```python
from build123d import *

# Parameters (mm, degrees)
F1_W          = 40
F1_H          = 40
F1_R          = 1.7
F2_DEPTH      = 3
F0_W          = 29.764212
F0_H          = 22.853858
F3_DEPTH      = 15
F0_W_2        = 24.935725
F0_H_2        = 6.393774
F4_DEPTH      = 3
F5_R          = 10
F7_DEPTH      = 25
F7_DEPTH_BACK = 25


with BuildPart() as f2:
    # F1 (on Front) → F2 (new body)
    with BuildSketch(Plane.XZ):
        Rectangle(F1_W, F1_H)
        with Locations((-16.410692, -16.77718)):
            Circle(F1_R, mode=Mode.SUBTRACT)
        with Locations((16.730379, -16.836943)):
            Circle(F1_R, mode=Mode.SUBTRACT)
        with Locations((-16.410692, 16.623817)):
            Circle(F1_R, mode=Mode.SUBTRACT)
        with BuildLine():
            ThreePointArc((-13.886995, 10.649008), (5.622615, 16.572151), (17.5, 0))
            ThreePointArc((17.5, 0), (5.622615, -16.572151), (-13.886995, -10.649008))
            ThreePointArc((-13.886995, -10.649008), (-17.5, 0), (-13.886995, 10.649008))
        make_face(mode=Mode.SUBTRACT)
        with Locations((16.31801, 16.738871)):
            Circle(F1_R, mode=Mode.SUBTRACT)
        with BuildLine():
            Line((-13.886995, -10.649008), (-13.886995, 10.649008))
            ThreePointArc((-13.886995, 10.649008), (-17.5, 0), (-13.886995, -10.649008))
        make_face()
    extrude(amount=F2_DEPTH)

    # F0 (on Front) → F3 (join)
    with BuildSketch(Plane.XZ):
        Polygon((19.911033, 13.426929), (-13.853179, 13.426929), (-13.853179, -13.426929), (-12.467862, -13.426929), (12.467863, -13.426929), (19.911033, -13.426929), align=None)
        with Locations((3.028927, 0)):
            Rectangle(F0_W, F0_H, mode=Mode.SUBTRACT)
    extrude(amount=F3_DEPTH)

    # F0 (on Front) → F4 (join)
    with BuildSketch(Plane.XZ):
        with Locations((0, -16.623816)):
            Rectangle(F0_W_2, F0_H_2)
    extrude(amount=F4_DEPTH)

    # F5 (on Top) → F7 (cut, two sides)
    with BuildSketch(Plane.XY) as f7_sk:
        with Locations((0, -18.9682)):
            Circle(F5_R)
    extrude(amount=F7_DEPTH, mode=Mode.SUBTRACT)
    extrude(f7_sk.sketch, amount=-F7_DEPTH_BACK, mode=Mode.SUBTRACT)


solid = f2.part
```
The model under review builds one solid part; all positions refer to its coordinate system, in mm. A direction names the side the tool comes from. Round coordinates to 2 decimals unless told otherwise and drop trailing zeros. Order: outer loops, then holes, each group sorted by start corner. A loop starts at its lowest first (then second) coordinate and runs counter-clockwise, first axis right, second up. Notation, with made-up numbers: (-33, 24) -> (-22, 24) arc R27 ccw to (-22, 45) -> close; hole circle Ø3 at (46.25, 9). An arc over 180 degrees is marked (long way). Use a Markdown table: item, result.
Q1. Mouldability with a two-part tool opening along Z and no side actions: class faces 1 (the flat face through (-11.853, -7, 0)), 2 (the flat face through (-13, -15, 0)), 3 (the flat face through (0, -1, 20)) as +Z half, -Z half, draft (parallel to the pull), parting line (faces both ways), or undercut.
Values:
| item | result |
|---|---|
| face 1 | undercut |
| face 2 | draft |
| face 3 | +Z half |
Q2. We need section D-D on x = -12.5. Write out the cut boundary in (y, z), then the cut area to 3 significant figures.
Values:
| item | result |
|---|---|
| outline | (-15, -13.43) -> (-3, -13.43) -> (-3, -20) -> (0, -20) -> (0, 20) -> (-3, 20) -> (-3, 13.43) -> (-15, 13.43) -> close |
| area | 442 mm^2 |
Q3. We need section A-A on y = -6. Write out the cut boundary in (x, z), then the cut area to 3 significant figures.
Values:
| item | result |
|---|---|
| outline | (-13.85, -13.43) -> (19.91, -13.43) -> (19.91, 13.43) -> (-13.85, 13.43) -> close; hole (-11.85, -11.43) -> (17.91, -11.43) -> (17.91, 11.43) -> (-11.85, 11.43) -> close |
| area | 226 mm^2 |
Q4. We need section C-C on z = 7. Write out the cut boundary in (x, y).
Values:
| item | result |
|---|---|
| outline | (-20, -3) -> (-13.89, -3) -> (-13.89, 0) -> (-20, 0) -> close; (-13.85, -15) -> (-11.85, -15) -> (-11.85, 0) -> (-13.85, 0) -> close; (16.04, -3) -> (17.91, -3) -> (17.91, -15) -> (19.91, -15) -> (19.91, -3) -> (20, -3) -> (20, 0) -> (16.04, 0) -> close |
Q5. Tool access review of faces 4 (the flat face through (3, -7, 13.427)), 5 (the cylindrical face through (15.065, -1.479, 17.888)), 6 (the flat face through (3, -8, -13.427)): name each direction out of +Z, -Z, +X, -X, +Y, -Y from which nothing blocks a thin tool from reaching the whole face with its end or side.
Values:
| item | result |
|---|---|
| face 4 | -Y |
| face 5 | +Y, -Y |
| face 6 | -Z, +X, -X, -Y |
Q6. Clearance check with flat-ended pins moving along their axes: P1, Ø8, axis at y = -5, z = 9, coming from the -X side; P2, Ø2.5, axis at x = 16.32, z = 16.74, coming from the +Y side; P3, Ø8, axis at x = 14, y = -13, coming from the +Z side; P4, Ø5, axis at y = -12, z = 10, coming from the +X side. State where each tip first meets the part, or that it passes through.
Values:
| item | result |
|---|---|
| P1 | stops at x = -20 |
| P2 | passes through |
| P3 | stops at z = 13.43 |
| P4 | stops at x = 19.91 |
Q7. For line 1 (X direction, y = -9.25, z = -1); line 2 (Z direction, x = -3, y = -0.75); line 3 (Z direction, x = 10, y = -11.75), list the stretches that pass through material, from the lowest coordinate up.
Values:
| item | result |
|---|---|
| line 1 | x = -13.85 to -11.85, 17.91 to 19.91 |
| line 2 | z = -20 to -11.43, 11.43 to 13.43, 17.24 to 20 |
| line 3 | z = -13.43 to -11.43, 11.43 to 13.43 |
Q8. We need section B-B on x = -4.5. Write out the cut boundary in (y, z).
Values:
| item | result |
|---|---|
| outline | (-10.04, -13.43) -> (-3, -13.43) -> (-3, -20) -> (0, -20) -> (0, -11.43) -> (-10.04, -11.43) -> close; (-10.04, 11.43) -> (0, 11.43) -> (0, 13.43) -> (-10.04, 13.43) -> close; (-3, 16.91) -> (0, 16.91) -> (0, 20) -> (-3, 20) -> close |
